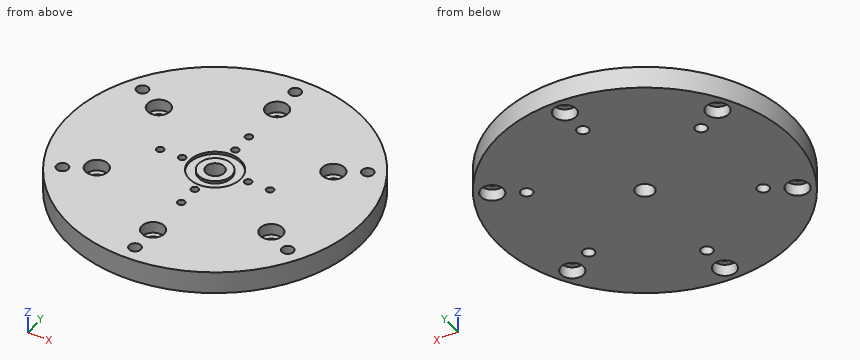
Solid Edge part; units mm, degrees
sketch "Sketch1" plane through (0, 0, 0) normal (0, 0, 1) x (1, 0, 0)
  circle A0 centre (0, 0) radius 40
extrude "Protrusion1" add sketch "Sketch1" along normal blind 6
sketch "Sketch2" plane through (0, 0, 6) normal (0, 0, 1) x (1, 0, 0)
  circle A0 centre (0, 27.5) radius 1.6
  circle A1 centre (0, 35.5) radius 1.6
extrude "Cutout1" cut sketch "Sketch2" against normal up to next
sketch "Sketch3" plane through (0, 0, 0) normal (0, 0, -1) x (1, 0, 0)
  circle A0 centre (0, -35.5) radius 3.05
extrude "ExtrudedCutout_2" cut sketch "Sketch3" against normal blind 3.2
sketch "Sketch4" plane through (0, 0, 6) normal (0, 0, 1) x (1, 0, 0)
  circle A0 centre (0, 27.5) radius 3.05
extrude "ExtrudedCutout_5" cut sketch "Sketch4" against normal blind 3.1
pattern_circular "Pattern1" count 6 over 360 about axis through (0, 0, 6) along (0, 0, -1) of "Cutout1", "ExtrudedCutout_2", "ExtrudedCutout_5"
sketch "Sketch5" plane through (0, 0, 6) normal (0, 0, 1) x (1, 0, 0)
  circle A0 centre (0, 0) radius 2.5
extrude "Cutout2" cut sketch "Sketch5" against normal up to next
sketch "Sketch6" plane through (0, 0, 6) normal (0, 0, 1) x (1, 0, 0)
  circle A0 centre (0, 0) radius 4.5
  circle A1 centre (0, 0) radius 7
extrude "ExtrudedCutout_4" cut sketch "Sketch6" against normal blind 0.7
hole "Hole_3" at (0, -9, 6) direction (0, 0, -1) diameter 2.013 depth 4.5 thread major 2.5 thread length 2
hole "Hole1" at (0, -15, 6) direction (0, 0, -1) diameter 2.013 depth 4.5 thread major 2.5 thread length 2
pattern_circular "Pattern4" count 4 over 360 about axis through (0, 0, 6) along (0, 0, 1) of "Hole_3", "Hole1"
CAD build for the part. Positions are in the model's coordinates, mm. Round coordinates to 2 decimals unless told otherwise and drop trailing zeros. Loops run counter-clockwise (first coordinate to the right, second up) from the corner with the lowest first, then second, coordinate; pieces in that order, holes last. Notation, with made-up numbers: M 78,-13 L 88,-13 A25 cw 88,22 Z; hole C -24,-33 d4. An arc over 180 degrees is marked long. Return JSON: item names as keys, results as strings. Group by question number.
(1) Drop flat-ended pins along their axis: P1, Ø1.8, axis at x = -1.5, y = 36.5, coming from the -Z side; P2, Ø3, axis at x = 0, y = 0, coming from the +Z side; P3, Ø1, axis at y = -30, z = 4, coming from the +X side; P4, Ø3, axis at x = -7.5, z = 4, coming from the -Y side. Give the stop position or say it passes through.
(2) Saw through at D-D, the plane y = 27.5. List the corners of the cut face in (x, z).
(3) Saw through at B-B, the plane x = 6. List the corners of the cut face in (y, z), and give its area (3 significant figures).
(4) Saw through at C-C, the plane y = 17.75. List the corners of the cut face in (x, z).
(5) Wall check: probe 1 along X at (y, z) = (-18, 0.45); probe 2 along Y at (x, z) = (29.5, 2.35); probe 3 along Y at (x, z) = (-25, 3.9). Give the ranges that are in metal, low to high. Write a range as [from, to].
Answer list:
{
 "1": {"P1": "z = 3.2", "P2": "through", "P3": "x = 27.01", "P4": "y = -39.55"},
 "2": {"outline": "M -29.05,0 L -1.6,0 L -1.6,2.9 L -3.05,2.9 L -3.05,6 L -29.05,6 Z; M 1.6,0 L 29.05,0 L 29.05,6 L 3.05,6 L 3.05,2.9 L 1.6,2.9 Z"},
 "3": {"outline": "M -39.55,0 L 39.55,0 L 39.55,6 L 3.61,6 L 3.61,5.3 L -3.61,5.3 L -3.61,6 L -39.55,6 Z", "area": "470 mm2"},
 "4": {"outline": "M -35.85,0 L -33.79,0 L -33.79,3.2 L -32.34,3.2 L -32.34,6 L -35.85,6 Z; M -29.14,3.2 L -27.69,3.2 L -27.69,0 L 27.69,0 L 27.69,3.2 L 29.14,3.2 L 29.14,6 L -29.14,6 Z; M 32.34,3.2 L 33.79,3.2 L 33.79,0 L 35.85,0 L 35.85,6 L 32.34,6 Z"},
 "5": {"probe 1": "[-35.72, -33.78], [-27.7, 27.7], [33.78, 35.72]", "probe 2": "[-27.01, -20.53], [-14.97, 14.97], [20.53, 27.01]", "probe 3": "[-31.22, -16.56], [-10.94, 10.94], [16.56, 31.22]"}
}
